Input: part model. Units: mm. Frame: model coordinates. A direction names the side the tool comes from. Give positions to 0.01 mm unless a question says otherwise; leave off trailing zeros. Loops run counter-clockwise (first coordinate to the right, second up) from the corner with the lowest first, then second, coordinate; pieces in that order, holes last. Notation, with made-up numbers: M 78.25,78 L 84.25,78 A30 ccw 84.25,114 Z; hole C -5,76 d11. An arc over 180 degrees is marked long. Use CSV: the item, a comma, the result in double quotes. Start each with the question number.
from build123d import *

# Parameters (mm, degrees)
SKETCH_1_W          = 40
SKETCH_1_H          = 50
EXTRUDE_1_DEPTH     = 8
SKETCH_2_W          = 3.2
SKETCH_2_H          = 4
CUT_EXTRUDE_1_DEPTH = 6.5
SKETCH_3_W          = 6
SKETCH_3_H          = 3
CUT_EXTRUDE_2_DEPTH = 16.5
SKETCH_10_R         = 1.6
CUT_EXTRUDE_7_DEPTH = 13
SKETCH_11_W         = 6
SKETCH_11_H         = 6
CUT_EXTRUDE_8_DEPTH = 3


with BuildPart() as part:
    # 草图1 → 凸台-拉伸1 (new body)
    with BuildSketch(Plane(origin=(0, 0, 0), x_dir=(1, 0, 0), z_dir=(0, 1, 0))):
        with Locations((20, 25)):
            Rectangle(SKETCH_1_W, SKETCH_1_H)
    extrude(amount=EXTRUDE_1_DEPTH)

    # 草图2 → 切除-拉伸1 (cut)
    with BuildSketch(Plane.XZ):
        with Locations((5, -2)):
            Rectangle(SKETCH_2_W, SKETCH_2_H)
        with Locations((15, -2)):
            Rectangle(SKETCH_2_W, SKETCH_2_H)
        with Locations((25, -2)):
            Rectangle(SKETCH_2_W, SKETCH_2_H)
        with Locations((35, -2)):
            Rectangle(SKETCH_2_W, SKETCH_2_H)
    extrude(amount=-CUT_EXTRUDE_1_DEPTH, mode=Mode.SUBTRACT)

    # 草图3 → 切除-拉伸2 (cut)
    with BuildSketch(Plane.XZ):
        with Locations((5, -5.5)):
            Rectangle(SKETCH_3_W, SKETCH_3_H)
        with Locations((15, -5.5)):
            Rectangle(SKETCH_3_W, SKETCH_3_H)
        with Locations((25, -5.5)):
            Rectangle(SKETCH_3_W, SKETCH_3_H)
        with Locations((35, -5.5)):
            Rectangle(SKETCH_3_W, SKETCH_3_H)
    extrude(amount=-CUT_EXTRUDE_2_DEPTH, mode=Mode.SUBTRACT)

    # 草图10 → 切除-拉伸7 (cut)
    with BuildSketch(Plane(origin=(0, 8, 0), x_dir=(1, 0, 0), z_dir=(0, 1, 0))):
        with Locations(Location((34, 16, 0), (0, 0, 270))):
            Circle(SKETCH_10_R)
        with Locations(Location((34, 26, 0), (0, 0, 270))):
            Circle(SKETCH_10_R)
        with Locations(Location((34, 36, 0), (0, 0, 270))):
            Circle(SKETCH_10_R)
    extrude(amount=-CUT_EXTRUDE_7_DEPTH, mode=Mode.SUBTRACT)

    # 草图11 → 切除-拉伸8 (cut)
    with BuildSketch(Plane.XZ):
        with Locations((34, -26)):
            Rectangle(SKETCH_11_W, SKETCH_11_H)
        with Locations((34, -36)):
            Rectangle(SKETCH_11_W, SKETCH_11_H)
        with Locations((34, -16)):
            Rectangle(SKETCH_11_W, SKETCH_11_H)
    extrude(amount=-CUT_EXTRUDE_8_DEPTH, mode=Mode.SUBTRACT)


solid = part.part
Item 1: Section B-B (x = 34). State how many separate pieces and enclosed holes the cut face has, then the cut area to 3 significant figures.
Item 2: Section C-C (z = -3). Output: boundary loops of the cut face in (x, y).
Item 3: Material intervals for line 1 (Z direction, x = 34, y = 0.75); line 2 (X direction, y = 5.6, z = -26); line 3 (X direction, y = 1.25, z = -25.5), sorted ascending.
Item 4: First-contact query: pin 1 Ø1.6 at (x, z) = (25, -3) entering from -Y; pin 2 Ø3 at (x, z) = (33.5, -15) entering from -Y; pin 3 Ø2.5 at (x, z) = (34, -26) entering from -Y. Flat tips, straight axial feed; report the tip coordinate or a pass-through.
Item 5: Section A-A (z = -26). Output: boundary loops of the cut face in (x, y).
Item 6: Mould query, pull axis X, two halves, no side actions, for faces 1 (the cylindrical face through (32.58, 5.54, -25.26)), 2 (the cylindrical face through (33.03, 5.54, -17.27)), 3 (the flat face through (40, 4, -25)). Classes: +X half, -X half, draft (parallel to the pull), parting line (faces both ways), or undercut.
Item 7: Set-up query: faces 4 (the flat face through (25, 4, -7)), 5 (the flat face through (33.4, 3, -2)), 6 (the flat face through (31, 1, -16)). Return all of +Z, -Z, +X, -X, +Y, -Y with unobstructed straight access to the full face (end or side cutting, diameter ignored); none if empty.
Recorded:
1,separate pieces,"5"
1,enclosed holes,"0"
1,area,"248 mm²"
2,outline,"M 0,0 L 3.4,0 L 3.4,6.5 L 6.6,6.5 L 6.6,0 L 13.4,0 L 13.4,6.5 L 16.6,6.5 L 16.6,0 L 23.4,0 L 23.4,6.5 L 26.6,6.5 L 26.6,0 L 33.4,0 L 33.4,6.5 L 36.6,6.5 L 36.6,0 L 40,0 L 40,8 L 0,8 Z"
3,line 1,"-50 to -39, -33 to -29, -23 to -19, -13 to -7"
3,line 2,"0 to 32.4, 35.6 to 40"
3,line 3,"0 to 31, 37 to 40"
4,pin 1,"y = 6.5"
4,pin 2,"y = 3"
4,pin 3,"through"
5,outline,"M 0,0 L 31,0 L 31,3 L 32.4,3 L 32.4,8 L 0,8 Z; M 35.6,3 L 37,3 L 37,0 L 40,0 L 40,8 L 35.6,8 Z"
6,face 1,"undercut"
6,face 2,"undercut"
6,face 3,"+X half"
7,face 4,"+Y, -Y"
7,face 5,"+Z, -Y"
7,face 6,"-Y"
